Read the model definition and answer for the solid it produces. Units are mm, in the model's axes. Coordinates: 2 decimals unless noted, no trailing zeros. Write each loop counter-clockwise with the first axis right and the second up, starting at its lowest first coordinate (ties: lowest second). Pieces come first, ordered by that corner, then holes. Notation, with made-up numbers: (-3, 14.5) -> (3, 14.5) arc R32 ccw to (3, 51.5) -> close; hole circle Ø2 at (-32.5, -12.5). An arc over 180 degrees is marked (long way). Answer in a Markdown table with one row per item. Add a question column.
Item 1: Straight lines are drawn through the part: line 1 (Y direction, x = 0, z = 69.05) (3 decimals); line 2 (Z direction, x = -6, y = -4); line 3 (Z direction, x = 7.5, y = -4.5). For each, find the intervals that lie inside material, in ascending order. Write a range as from..to.
Item 2: Section B-B on x = 6 is taken. Write down the section's boundary in (y, z), then the cut area to 3 significant figures.
Item 3: Section C-C on z = 44.5 is taken. Write down the section's boundary in (x, y) (3 decimals).
Item 4: Section D-D on x = -3.25 is taken. Write down the section's boundary in (y, z).
Item 5: Given pin 1 Ø1 at (x, z) = (8.5, 47) entering from -Y; pin 2 Ø5 at (y, z) = (5.5, 32.5) entering from +X; pin 3 Ø1.5 at (y, z) = (-6, 24) entering from -X, each flat-ended and moving along its own axis, determine where each tip first touches the part or whether it passes through.
Item 6: Section A-A on y = 7 is taken. Write down the section's boundary in (x, z).
```python
from build123d import *

# Parameters (mm, degrees)
SKETCH1_R           = 10.775
BOSS_EXTRUDE1_DEPTH = 68.45
SKETCH2_R           = 4.7
BOSS_EXTRUDE2_DEPTH = 1.7
SKETCH3_R           = 10.5
SKETCH3_R_2         = 8.275
BOSS_EXTRUDE3_DEPTH = 0.8


with BuildPart() as part:
    # Sketch1 → Boss-Extrude1 (new body)
    with BuildSketch(Plane.XY):
        Circle(SKETCH1_R)
    extrude(amount=BOSS_EXTRUDE1_DEPTH)

    # Sketch2 → Boss-Extrude2 (add)
    with BuildSketch(Plane.XY.offset(68.45)):
        Circle(SKETCH2_R)
    extrude(amount=BOSS_EXTRUDE2_DEPTH)

    # Sketch3 → Boss-Extrude3 (add)
    with BuildSketch(Plane.XY.offset(68.45)):
        Circle(SKETCH3_R)
        Circle(SKETCH3_R_2, mode=Mode.SUBTRACT)
    extrude(amount=BOSS_EXTRUDE3_DEPTH)


solid = part.part
```
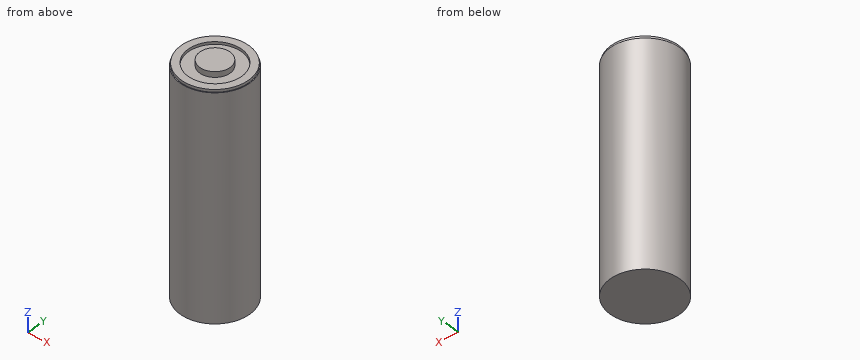
Results below:
| question | item | result |
|---|---|---|
| 1 | line 1 | y = -10.5..-8.275, -4.7..4.7, 8.275..10.5 |
| 1 | line 2 | z = 0..68.45 |
| 1 | line 3 | z = 0..69.25 |
| 2 | outline | (-8.95, 0) -> (8.95, 0) -> (8.95, 68.45) -> (8.62, 68.45) -> (8.62, 69.25) -> (5.7, 69.25) -> (5.7, 68.45) -> (-5.7, 68.45) -> (-5.7, 69.25) -> (-8.62, 69.25) -> (-8.62, 68.45) -> (-8.95, 68.45) -> close |
| 2 | area | 1,230 mm2 |
| 3 | outline | circle Ø21.55 at (0, 0) |
| 4 | outline | (-10.27, 0) -> (10.27, 0) -> (10.27, 68.45) -> (9.98, 68.45) -> (9.98, 69.25) -> (7.61, 69.25) -> (7.61, 68.45) -> (3.4, 68.45) -> (3.4, 70.15) -> (-3.4, 70.15) -> (-3.4, 68.45) -> (-7.61, 68.45) -> (-7.61, 69.25) -> (-9.98, 69.25) -> (-9.98, 68.45) -> (-10.27, 68.45) -> close |
| 5 | pin 1 | stops at y = -7.22 |
| 5 | pin 2 | stops at x = 10.35 |
| 5 | pin 3 | stops at x = -9.41 |
| 6 | outline | (-8.19, 0) -> (8.19, 0) -> (8.19, 68.45) -> (7.83, 68.45) -> (7.83, 69.25) -> (4.41, 69.25) -> (4.41, 68.45) -> (-4.41, 68.45) -> (-4.41, 69.25) -> (-7.83, 69.25) -> (-7.83, 68.45) -> (-8.19, 68.45) -> close |
